Check sheet for the drawn part. Datum: minimum x, y, z corner. Units: mm. A direction names the side the tool comes from. Round coordinates to 2 decimals unless told otherwise and drop trailing zeros. Write each loop counter-clockwise with the first axis right and the second up, starting at its lowest first coordinate (ties: lowest second). Pieces come first, ordered by that corner, then holes. Notation, with made-up numbers: (-11.75, 70.5) - (11.25, 70.5) arc R17 ccw to (11.25, 78.5) - close; hole circle Ø1 at (79.5, -22.5). An arc over 180 degrees is marked (long way). Answer as a JSON object with one key per item and string values. Group by question number.
1) Section check D-D (z = 16). Enter the section's corners in (x, y), then the cut area to 3 significant figures.
2) Thickness scan on line 1 (Z direction, x = 1.75, y = 11.75); line 2 (X direction, y = 12, z = 19). Record the ranges inside material, lowest first.
3) Set-up check for the marked faces 1, 2 and 3: record each of +Z, -Z, +X, -X, +Y, -Y from which the full face is reachable in a straight line by a thin tool's end or side.
4) Section check C-C (x = 8). Enter the section's corners in (y, z).
5) Section check B-B (y = 8). Enter the section's corners in (x, z).
6) Go/stop test with flat-tipped pins: pin 1 Ø1 at (y, z) = (2, 17.5) entering from -X; pin 2 Ø0.5 at (x, z) = (1, 0.5) entering from +Y; pin 3 Ø0.5 at (y, z) = (15, 0.5) entering from +X; pin 4 Ø0.8 at (y, z) = (15, 0.5) entering from -X. Record where each tip stops, or that it passes through.
7) Section check A-A (z = 12). Enter the section's corners in (x, y), then the cut area to 3 significant figures.
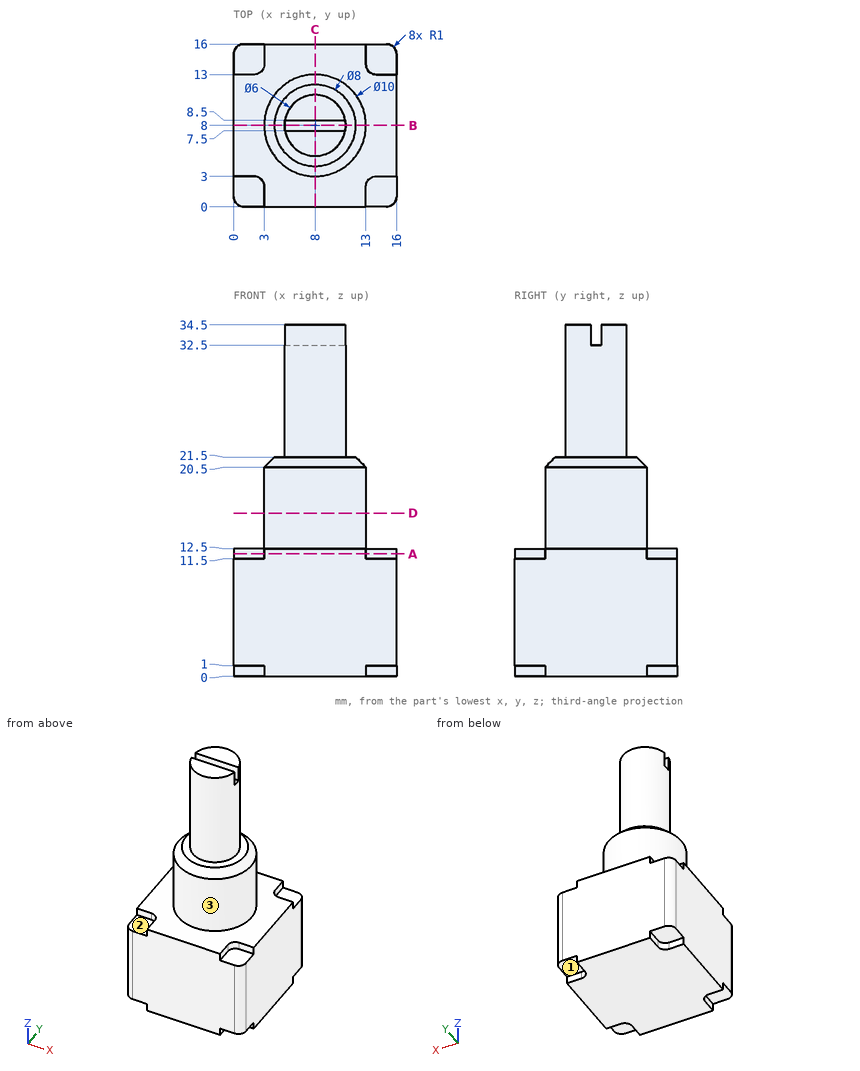
Returned:
{
 "1": {"outline": "circle Ø10 at (8, 8)", "area": "78.5 mm2"},
 "2": {"line 1": "0 to 12.5", "line 2": "5 to 11"},
 "3": {"face 1": "-Z, +X, +Y", "face 2": "+Z, -X, -Y", "face 3": "+Z"},
 "4": {"outline": "(0, 0) - (16, 0) - (16, 12.5) - (13, 12.5) - (13, 20.5) - (12, 21.5) - (11, 21.5) - (11, 34.5) - (8.5, 34.5) - (8.5, 32.5) - (7.5, 32.5) - (7.5, 34.5) - (5, 34.5) - (5, 21.5) - (4, 21.5) - (3, 20.5) - (3, 12.5) - (0, 12.5) - close"},
 "5": {"outline": "(0, 0) - (16, 0) - (16, 12.5) - (13, 12.5) - (13, 20.5) - (12, 21.5) - (11, 21.5) - (11, 32.5) - (5, 32.5) - (5, 21.5) - (4, 21.5) - (3, 20.5) - (3, 12.5) - (0, 12.5) - close"},
 "6": {"pin 1": "through", "pin 2": "y = 13", "pin 3": "x = 13", "pin 4": "x = 3"},
 "7": {"outline": "(0, 3) - (2, 3) arc R1 cw to (3, 2) - (3, 0) - (13, 0) - (13, 2) arc R1 cw to (14, 3) - (16, 3) - (16, 13) - (14, 13) arc R1 cw to (13, 14) - (13, 16) - (3, 16) - (3, 14) arc R1 cw to (2, 13) - (0, 13) - close", "area": "221 mm2"}
}
